Geometry: final body of the model. Coordinates: model frame, mm. A direction names the side the tool comes from. Give positions to 0.01 mm unless a question says otherwise; leave off trailing zeros. Write each loop counter-clockwise with the first axis right and the second up, starting at its lowest first coordinate (ties: lowest second). Pieces come first, ordered by that corner, then holes.
```python
from build123d import *

# Parameters (mm, degrees)
SKETCH_1_W             = 25.7
SKETCH_1_H             = 36
EXTRUDE_1_DEPTH        = 1.56
SKETCH_2_R             = 1.5
CUT_EXTRUDE_1_DEPTH    = 1.56
SKETCH_3_W             = 2.54
SKETCH_3_H             = 2.54
EXTRUDE_2_DEPTH        = 2.5
CHAMFER_1_SIZE         = 0.3
PATTERN_START          = 1.56
PATTERN_LINEAR_1_DEPTH = 2.5
SKETCH_4_W             = 15
SKETCH_4_H             = 12
EXTRUDE_3_DEPTH        = 2.5
SKETCH_5_W             = 0.664657546
SKETCH_5_H             = 0.664657545
EXTRUDE_4_DEPTH        = 3
PATTERN_LINEAR_2_COUNT = 4
PATTERN_LINEAR_2_PITCH = 2.54


# Read off the part's stored shape, not the designer's step: 阵列(线性)1
with BuildPart() as part:
    # 草图1 → 凸台-拉伸1 (new body)
    with BuildSketch(Plane(origin=(0, 0, 0), x_dir=(0, 0, -1), z_dir=(1, 0, 0))):
        Rectangle(SKETCH_1_W, SKETCH_1_H)
    extrude(amount=EXTRUDE_1_DEPTH)

    # 草图2 → 切除-拉伸1 (cut)
    with BuildSketch(Plane(origin=(1.56, 0, 0), x_dir=(0, 0, -1), z_dir=(1, 0, 0))):
        with Locations((-10.35, 15.5)):
            Circle(SKETCH_2_R)
        with Locations((10.35, 15.5)):
            Circle(SKETCH_2_R)
        with Locations((-10.35, -15.5)):
            Circle(SKETCH_2_R)
        with Locations((10.35, -15.5)):
            Circle(SKETCH_2_R)
    extrude(amount=-CUT_EXTRUDE_1_DEPTH, mode=Mode.SUBTRACT)

    # 草图3 → 凸台-拉伸2 (add)
    with BuildSketch(Plane(origin=(1.56, 0, 0), x_dir=(0, 0, -1), z_dir=(1, 0, 0))):
        with Locations((-3.81, -16.609886397)):
            Rectangle(SKETCH_3_W, SKETCH_3_H)
    extrude(amount=EXTRUDE_2_DEPTH)

    # 倒角1
    chamfer_1_edges = [part.edges().sort_by_distance(p)[0] for p in [
        (2.81, -17.879886397, 2.54),
        (2.81, -15.339886397, 2.54),
        (2.81, -15.339886397, 5.08),
        (2.81, -17.879886397, 5.08),
    ]]
    chamfer(chamfer_1_edges, length=CHAMFER_1_SIZE)

    # 阵列(线性)1 outline → 阵列(线性)1 (add)
    with BuildSketch(Plane.YZ.offset(PATTERN_START)):
        Polygon((-15.339886397, 0.3), (-15.339886397, 2.24), (-15.639886397, 2.54), (-17.579886397, 2.54), (-17.879886397, 2.24), (-17.879886397, 0.3), (-17.579886397, 0), (-17.879886397, -0.3), (-17.879886397, -2.24), (-17.579886397, -2.54), (-17.879886397, -2.84), (-17.879886397, -4.78), (-17.579886397, -5.08), (-15.639886397, -5.08), (-15.339886397, -4.78), (-15.339886397, -2.84), (-15.639886397, -2.54), (-15.339886397, -2.24), (-15.339886397, -0.3), (-15.639886397, 0), align=None)
    extrude(amount=PATTERN_LINEAR_1_DEPTH)

    # 草图4 → 凸台-拉伸3 (add)
    with BuildSketch(Plane(origin=(1.56, 0, 0), x_dir=(0, 0, -1), z_dir=(1, 0, 0))):
        with Locations((-0.05, 0.52)):
            Rectangle(SKETCH_4_W, SKETCH_4_H)
    extrude(amount=EXTRUDE_3_DEPTH)

    # 草图5 → 凸台-拉伸4 (add)
    with BuildSketch(Plane(origin=(4.06, 0, 0), x_dir=(0, 0, -1), z_dir=(1, 0, 0))):
        with Locations((-3.81, -16.609886397)):
            Rectangle(SKETCH_5_W, SKETCH_5_H)
    extrude_4 = extrude(amount=EXTRUDE_4_DEPTH)

    # 阵列(线性)2: 凸台-拉伸4 ×4
    with Locations(*[(0, 0, -i * PATTERN_LINEAR_2_PITCH) for i in range(1, PATTERN_LINEAR_2_COUNT)]):
        add(extrude_4)


solid = part.part
```
Item 1: Section C-C, the plane z = 10.35. Return the cut outline in (x, y), plus the area to 3 significant figures.
Found:
outline: (0, -18) - (1.56, -18) - (1.56, -17) - (0, -17) - close; (0, -14) - (1.56, -14) - (1.56, 14) - (0, 14) - close; (0, 17) - (1.56, 17) - (1.56, 18) - (0, 18) - close
area: 46.8 mm2
Item 2: Pull-direction query (Y, two-part tool) for faces 1 (the face through (4.06, -17, 0)), 2 (the face through (3, -5.48, 0)), 3 (the face through (1, 18, 0)); classes: +Y half, -Y half, draft (parallel to the pull), parting line (faces both ways), or undercut.
Found:
face 1: draft
face 2: undercut
face 3: +Y half
Item 3: Section A-A, the plane y = 15.5. Return the cut outline in (x, z).
Found:
outline: (0, -12.85) - (1.56, -12.85) - (1.56, -11.85) - (0, -11.85) - close; (0, -8.85) - (1.56, -8.85) - (1.56, 8.85) - (0, 8.85) - close; (0, 11.85) - (1.56, 11.85) - (1.56, 12.85) - (0, 12.85) - close
Item 4: Pin query (flat end, axial travel): pin 1 Ø2.5 at (y, z) = (15.5, 10.35) entering from +X; pin 2 Ø0.8 at (x, z) = (2.5, -2) entering from -Y; pin 3 Ø1 at (y, z) = (-1.5, 3.5) entering from +X; pin 4 Ø2 at (x, z) = (2.5, -2.5) entering from +Y. Return the tip coordinate at first contact, or that it passes through.
Found:
pin 1: passes through
pin 2: stops at y = -17.88
pin 3: stops at x = 4.06
pin 4: stops at y = 18
Item 5: Line query: L1, parallel to Y at x = 0.65, z = 10.35; L2, parallel to X at y = -12.5, z = -6; L3, parallel to Y at x = 2, z = -7.25. Output: solid intervals per line, ascending.
Found:
L1: y = -18 to -17, -14 to 14, 17 to 18
L2: x = 0 to 1.56
L3: y = -5.48 to 6.52
Item 6: Reachability of faces 4 (the face through (4.06, 1, 0)), 5 (the face through (3, 0, 7.55)), 6 (the face through (3, 0, -7.45)), 7 (the face through (3, -15.34, -4)), 8 (the face through (3, -17.88, -4)) from +Z, -Z, +X, -X, +Y, -Y: full face, straight path, thin tool, end or side. Return the list, or none.
Found:
face 4: +Z, -Z, +X, +Y
face 5: +Z, +X, +Y, -Y
face 6: -Z, +X, +Y, -Y
face 7: +Z, -Z, +X
face 8: +Z, -Z, +X, -Y
Item 7: Section D-D, the plane x = 5.5. Return the cut outline in (y, z).
Found:
outline: (-16.94, -4.14) - (-16.28, -4.14) - (-16.28, -3.48) - (-16.94, -3.48) - close; (-16.94, -1.6) - (-16.28, -1.6) - (-16.28, -0.94) - (-16.94, -0.94) - close; (-16.94, 0.94) - (-16.28, 0.94) - (-16.28, 1.6) - (-16.94, 1.6) - close; (-16.94, 3.48) - (-16.28, 3.48) - (-16.28, 4.14) - (-16.94, 4.14) - close
